Could you check a few things on this model? Use its own coordinates, in mm. A direction names the side the tool comes from. Round coordinates to 2 decimals unless told otherwise and drop trailing zeros. Order: outer loops, then holes, each group sorted by start corner. A loop starts at its lowest first (then second) coordinate and runs counter-clockwise, first axis right, second up. Notation, with made-up numbers: M 32.5,-5 L 87.5,-5 A7 cw 87.5,0 Z; hole C 28.25,10 d2. An arc over 180 degrees is marked long. Write each question's results on one line, items separated by ' | '. Start each with the question number.
1. Suppose I cut it at A-A on y = -15. Write out the boundary of the cut face in (x, z).
2. Please list where these lines run through material, in increasing order: L1, parallel to X at y = -15, z = 2.7; L2, parallel to Y at x = 44.75, z = 5; L3, parallel to X at y = -3.25, z = 8.5.
3. Suppose I cut it at D-D on y = -3. Give the number of separate pieces and of enclosed holes in the cut face, and give its area (4 significant figures).
4. For faces 4 (the flat face through (7, -3, 2)), 5 (the cylindrical face through (10.02, -4.15, 11.99)), 6 (the cylindrical face through (24.254, -16.339, 2.958)), 7 (the flat face through (18.5, -15, 4)), which set-ups out of +Z, -Z, +X, -X, +Y, -Y let a thin tool reach every point of the face, with its end or its side?
5. I'm going to push flat-ended pins straight in: pin 1 (11 mm diameter, centred on x = 16.5, y = -9, fed in from +Z); pin 2 (7 mm diameter, centred on y = -17, z = 6, fed in from -X); pin 3 (7 mm diameter, centred on x = 47.5, z = 3.5, fed in from -Y). Where does each tip first touch, or does it pass through?
6. We'd pull the mould along X, two halves only. Please class faces 1 (the flat face through (17.3, -8.8, 4.4)), 2 (the flat face through (33.5, -15, 4)), 3 (the cylindrical face through (9.635, -2.249, 9.74)): released by +X, released by -X, zero draft, split by the parting line, or undercut.
7. Suppose I cut it at B-B on z = 5.5. Write out the boundary of the cut face in (x, y).
from build123d import *

# Parameters (mm, degrees)
SKETCH1_W                = 52
SKETCH1_H                = 7.5
SKETCH1_R                = 2.5
SKETCH1_W_2              = 15
SKETCH1_H_2              = 15
SKETCH1_R_2              = 2.2
BOSS_EXTRUDE1_DEPTH      = 9
BOSS_EXTRUDE2_DEPTH      = 1.5
BOSS_EXTRUDE2_DEPTH_BACK = 9
SKETCH2_R                = 2.5
SKETCH4_R                = 3
BOSS_EXTRUDE3_DEPTH      = 2.5
CHAMFER1_SIZE            = 0.5
CHAMFER2_SIZE            = 2.5
CUT_EXTRUDE1_DEPTH       = 2
CUT_EXTRUDE1_DEPTH_BACK  = 7
SKETCH5_R                = 1.25


with BuildPart() as part:
    # Sketch1 → Boss-Extrude1 (new body)
    # profile 1 of 2: a face of its own
    with BuildSketch(Plane.XY):
        with Locations((26, -3.75)):
            Rectangle(SKETCH1_W, SKETCH1_H)
        with Locations((7.25, -3)):
            Circle(SKETCH1_R, mode=Mode.SUBTRACT)
        with Locations((44.75, -3)):
            Circle(SKETCH1_R, mode=Mode.SUBTRACT)
    # profile 2 of 2: a face of its own
    with BuildSketch(Plane.XY):
        with Locations((26, -15)):
            Rectangle(SKETCH1_W_2, SKETCH1_H_2)
        with Locations((26, -15)):
            Circle(SKETCH1_R_2, mode=Mode.SUBTRACT)
    extrude(amount=BOSS_EXTRUDE1_DEPTH)

    # Sketch2 → Boss-Extrude2 (add, two sides: drawn at the far end of the back side and taken through both)
    with BuildSketch(Plane.XY.offset(9).offset(-BOSS_EXTRUDE2_DEPTH_BACK)):
        with Locations((7.25, -3)):
            Circle(SKETCH2_R)
        with Locations((44.75, -3)):
            Circle(SKETCH2_R)
    extrude(amount=BOSS_EXTRUDE2_DEPTH + BOSS_EXTRUDE2_DEPTH_BACK)

    # Sketch3 → Cut-Revolve1 (revolve, cut)
    with BuildSketch(Plane(origin=(0, -15, 0), x_dir=(1, 0, 0), z_dir=(0, 1, 0)), mode=Mode.PRIVATE) as cut_revolve1_sk:
        Polygon((26, -9), (30.807860213, -9), (28.2, -6), (26, -6), align=None)
    revolve(cut_revolve1_sk.sketch.rotate(Axis((26, -15, 6), (0, 0, 1)), 180), axis=Axis((26, -15, 6), (0, 0, 1)), mode=Mode.SUBTRACT)

    # Sketch4 → Boss-Extrude3 (add)
    with BuildSketch(Plane.XY.offset(10.5)):
        with Locations((7.25, -3)):
            Circle(SKETCH4_R)
        with Locations((44.75, -3)):
            Circle(SKETCH4_R)
    extrude(amount=BOSS_EXTRUDE3_DEPTH)

    # Chamfer1
    chamfer1_edges = [part.edges().sort_by_distance(p)[0] for p in [
        (4.25, -3, 10.5),
        (41.75, -3, 10.5),
    ]]
    chamfer(chamfer1_edges, length=CHAMFER1_SIZE - 0.0001)  # a hair under: the kernel refuses the full size

    # Chamfer2
    chamfer2_edges = [part.edges().sort_by_distance(p)[0] for p in [
        (33.5, -7.5, 4.5),
        (33.5, -22.5, 4.5),
        (18.5, -22.5, 4.5),
        (18.5, -7.5, 4.5),
    ]]
    chamfer(chamfer2_edges, length=CHAMFER2_SIZE)

    # Sketch5 → Cut-Extrude1 (cut, two sides: drawn at the far end of the back side and taken through both)
    with BuildSketch(Plane.XY.offset(9).offset(-CUT_EXTRUDE1_DEPTH_BACK)):
        with Locations((7.25, -3)):
            Circle(SKETCH5_R)
        with Locations((44.75, -3)):
            Circle(SKETCH5_R)
    extrude(amount=CUT_EXTRUDE1_DEPTH + CUT_EXTRUDE1_DEPTH_BACK, mode=Mode.SUBTRACT)


solid = part.part
Filled sheet:
1) outline: M 18.5,0 L 23.8,0 L 23.8,6 L 21.19,9 L 18.5,9 Z; M 28.2,0 L 33.5,0 L 33.5,9 L 30.81,9 L 28.2,6 Z
2) L1: x = 18.5 to 23.8, 28.2 to 33.5 | L2: y = -7.5 to -4.25, -1.75 to 0 | L3: x = 0 to 6.03, 8.47 to 43.53, 45.97 to 52
3) separate pieces: 1 | enclosed holes: 2 | area: 467.5 mm^2
4) face 4: none | face 5: +Z | face 6: +Z, -Z | face 7: +Z, -Z, -X, -Y
5) pin 1: stops at z = 9 | pin 2: stops at x = 18.5 | pin 3: stops at y = -7.5
6) face 1: released by -X | face 2: released by +X | face 3: undercut
7) outline: M 0,-7.5 L 16,-7.5 L 18.5,-10 L 18.5,-20 L 21,-22.5 L 31,-22.5 L 33.5,-20 L 33.5,-10 L 36,-7.5 L 52,-7.5 L 52,0 L 0,0 Z; hole C 7.25,-3 d2.5; hole C 26,-15 d4.4; hole C 44.75,-3 d2.5
